Verification items for the finished model (mm, model axes). A direction names the side the tool comes from. Give positions to 0.01 mm unless a question says otherwise; leave off trailing zeros. Write each loop counter-clockwise with the first axis right and the second up, starting at its lowest first coordinate (ties: lowest second). Pieces come first, ordered by that corner, then holes. Notation, with made-up numbers: (23.5, 69.5) -> (27.5, 69.5) arc R10 ccw to (27.5, 83.5) -> close; hole circle Ø9 at (89, -13.75). An arc over 180 degrees is marked (long way). Write item = value, one per line.
from build123d import *

# Parameters (mm, degrees)
GUIDE_RODS_DEPTH   = 25.4
GUIDE_RODS_2_DEPTH = 25.4
SKETCH2_W          = 181.102
SKETCH2_H          = 76.2
BASEPLATE_DEPTH    = 3.81
ROD_CUP_DEPTH      = 181.102
HANDLES_DEPTH      = 154.034720609


with BuildPart() as part:
    # Sketch1 → Guide rods (new body)
    with BuildSketch(Plane(origin=(0, 0, 0), x_dir=(1, 0, 0), z_dir=(0, 1, 0))):
        Polygon((-5.842, 0), (-7.112, -1.244340789), (-7.112, -8.610340789), (1.27, -8.610340789), (1.27, -1.244340789), (0, 0), align=None)
    extrude(amount=GUIDE_RODS_DEPTH)



with BuildPart() as body_2:
    # Sketch1 → Guide rods 2 (new body)
    with BuildSketch(Plane(origin=(0, 0, 0), x_dir=(1, 0, 0), z_dir=(0, 1, 0))):
        Polygon((90.678, 0), (89.408, -1.244340789), (89.408, -8.610340789), (97.79, -8.610340789), (97.79, -1.244340789), (96.52, 0), align=None)
    extrude(amount=GUIDE_RODS_2_DEPTH)


with BuildPart() as part_1:
    add(part.part)

    add(body_2.part)  # baseplate merges body 2
    # Sketch2 → baseplate (add)
    with BuildSketch(Plane(origin=(0, 25.4, 0), x_dir=(1, 0, 0), z_dir=(0, 1, 0))):
        with Locations((45.339, 25.933659211)):
            Rectangle(SKETCH2_W, SKETCH2_H)
    extrude(amount=BASEPLATE_DEPTH)

    # Sketch3 → rod cup (add)
    with BuildSketch(Plane.ZY.offset(45.212)):
        with BuildLine():
            Line((-48.370526129, 25.4), (-0.263262521, 25.4))
            Line((-0.263262521, 25.4), (-0.263262521, 10.48765464))
            Line((-0.263262521, 10.48765464), (-19.456659211, 10.48765464))
            ThreePointArc((-19.456659211, 10.48765464), (-24.663659211, 15.69465464), (-29.870659211, 10.48765464))
            Line((-29.870659211, 10.48765464), (-48.370526129, 10.48765464))
            Line((-48.370526129, 10.48765464), (-48.370526129, 25.4))
        make_face()
    extrude(amount=-ROD_CUP_DEPTH)

    # Sketch4 → Handles (cut, through all)
    with BuildSketch(Plane(origin=(0, 29.21, 0), x_dir=(1, 0, 0), z_dir=(0, 1, 0))):
        with BuildLine():
            Line((-13.462, 48.793659211), (-13.462, 3.073659211))
            ThreePointArc((-13.462, 3.073659211), (-26.162, -9.626340789), (-38.862, 3.073659211))
            Line((-38.862, 3.073659211), (-38.862, 48.793659211))
            ThreePointArc((-38.862, 48.793659211), (-26.162, 61.493659211), (-13.462, 48.793659211))
        make_face()
        with BuildLine():
            Line((104.14, 48.793659211), (104.14, 3.073659211))
            ThreePointArc((104.14, 3.073659211), (116.84, -9.626340789), (129.54, 3.073659211))
            Line((129.54, 3.073659211), (129.54, 48.793659211))
            ThreePointArc((129.54, 48.793659211), (116.84, 61.493659211), (104.14, 48.793659211))
        make_face()
    extrude(amount=-HANDLES_DEPTH, mode=Mode.SUBTRACT)


solid = part_1.part
Item 1: Go/stop test with flat-tipped pins: P1, Ø9.5, axis at x = 26.5, z = -7, coming from the -Y side; P2, Ø6, axis at x = -18, z = -20, coming from the +Y side; P3, Ø1.9, axis at x = 131.5, y = 17.5, coming from the -Z side; P4, Ø10, axis at x = 62, z = 5, coming from the -Y side. Record where each tip stops, or that it passes through.
Response values:
P1 = 10.49
P2 = through
P3 = -48.37
P4 = 25.4
Item 2: Material ranges on line 1 (X direction, y = 16.5, z = -43.5); line 2 (Z direction, x = -11.5, y = 10.75); line 3 (Y direction, x = 62, z = -35.5), recorded low to high.
Response values:
line_1 = -45.21 to -38.86, -13.46 to 104.14, 129.54 to 135.89
line_2 = -48.37 to -29.86, -19.46 to -0.26
line_3 = 10.49 to 29.21
Item 3: Mould release check, pull along Z, two halves, no side actions. Record for faces 4 (the flat face through (-42, 18, -48.371)), 5 (the flat face through (133, 10.488, -39)), 6 (the flat face through (129.54, 20, -26)): +Z half, -Z half, draft (parallel to the pull), parting line (faces both ways), or undercut.
Response values:
face_4 = -Z half
face_5 = draft
face_6 = undercut
Item 4: Sectioned sample at C-C on z = -52. Record the cut outline in (x, y), then the cut area to 3 significant figures.
Response values:
outline = (-45.21, 25.4) -> (-38.45, 25.4) -> (-38.45, 29.21) -> (-45.21, 29.21) -> close; (-13.87, 25.4) -> (104.55, 25.4) -> (104.55, 29.21) -> (-13.87, 29.21) -> close; (129.13, 25.4) -> (135.89, 25.4) -> (135.89, 29.21) -> (129.13, 29.21) -> close
area = 503 mm^2
Item 5: Sectioned sample at D-D on x = 17. Record the cut outline in (y, z).
Response values:
outline = (10.49, -48.37) -> (25.4, -48.37) -> (25.4, -64.03) -> (29.21, -64.03) -> (29.21, 12.17) -> (25.4, 12.17) -> (25.4, -0.26) -> (10.49, -0.26) -> (10.49, -19.46) arc R5.21 cw to (10.49, -29.87) -> close
Item 6: Sectioned sample at A-A on x = 116.84. Record the cut outline in (y, z), then the cut area to 3 significant figures.
Response values:
outline = (25.4, -64.03) -> (29.21, -64.03) -> (29.21, -61.49) -> (25.4, -61.49) -> close; (25.4, 9.63) -> (29.21, 9.63) -> (29.21, 12.17) -> (25.4, 12.17) -> close
area = 19.4 mm^2
Item 7: Sectioned sample at B-B on y = 23. Record the cut outline in (x, z).
Response values:
outline = (-45.21, -48.37) -> (-38.86, -48.37) -> (-38.86, -3.07) arc R12.7 cw to (-38.55, -0.26) -> (-45.21, -0.26) -> close; (-13.78, -0.26) arc R12.7 cw to (-13.46, -3.07) -> (-13.46, -48.37) -> (104.14, -48.37) -> (104.14, -3.07) arc R12.7 cw to (104.45, -0.26) -> close; (-7.11, 1.24) -> (-5.84, 0) -> (0, 0) -> (1.27, 1.24) -> (1.27, 8.61) -> (-7.11, 8.61) -> close; (89.41, 1.24) -> (90.68, 0) -> (96.52, 0) -> (97.79, 1.24) -> (97.79, 8.61) -> (89.41, 8.61) -> close; (129.23, -0.26) arc R12.7 cw to (129.54, -3.07) -> (129.54, -48.37) -> (135.89, -48.37) -> (135.89, -0.26) -> close
Item 8: Set-up check for faces 1 (the cylindrical face through (-25.883, 26.221, 9.623)), 2 (the flat face through (-42, 18, -0.263)), 3 (the flat face through (89.408, 13, 5)): record each of +Z, -Z, +X, -X, +Y, -Y from which the full face is reachable in a straight line by a thin tool's end or side.
Response values:
face_1 = +Y, -Y
face_2 = +Z, +X, -X, -Y
face_3 = +Z, -Y
